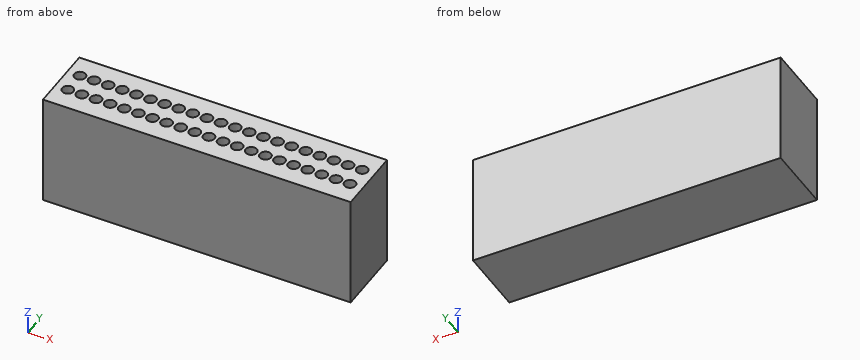
```python
from build123d import *

# Parameters (mm, degrees)
SKETCH2_W           = 27.25
SKETCH2_H           = 6
BOSS_EXTRUDE1_DEPTH = 10
SKETCH3_R           = 0.5
CUT_EXTRUDE1_DEPTH  = 5


with BuildPart() as part:
    # Sketch2 → Boss-Extrude1 (new body)
    with BuildSketch(Plane.XY):
        with Locations((13.625, 3)):
            Rectangle(SKETCH2_W, SKETCH2_H)
    extrude(amount=BOSS_EXTRUDE1_DEPTH)

    # Sketch3 → Cut-Extrude1 (cut)
    with BuildSketch(Plane.XY.offset(10)):
        with Locations((1.125, 2)):
            Circle(SKETCH3_R)
        with Locations((2.375, 2)):
            Circle(SKETCH3_R)
        with Locations((3.625, 2)):
            Circle(SKETCH3_R)
        with Locations((4.875, 2)):
            Circle(SKETCH3_R)
        with Locations((6.125, 2)):
            Circle(SKETCH3_R)
        with Locations((7.375, 2)):
            Circle(SKETCH3_R)
        with Locations((8.625, 2)):
            Circle(SKETCH3_R)
        with Locations((9.875, 2)):
            Circle(SKETCH3_R)
        with Locations((11.125, 2)):
            Circle(SKETCH3_R)
        with Locations((12.375, 2)):
            Circle(SKETCH3_R)
        with Locations((13.625, 2)):
            Circle(SKETCH3_R)
        with Locations((14.875, 2)):
            Circle(SKETCH3_R)
        with Locations((16.125, 2)):
            Circle(SKETCH3_R)
        with Locations((17.375, 2)):
            Circle(SKETCH3_R)
        with Locations((18.625, 2)):
            Circle(SKETCH3_R)
        with Locations((19.875, 2)):
            Circle(SKETCH3_R)
        with Locations((21.125, 2)):
            Circle(SKETCH3_R)
        with Locations((22.375, 2)):
            Circle(SKETCH3_R)
        with Locations((23.625, 2)):
            Circle(SKETCH3_R)
        with Locations((24.875, 2)):
            Circle(SKETCH3_R)
        with Locations((26.125, 2)):
            Circle(SKETCH3_R)
    cut_extrude1 = extrude(amount=-CUT_EXTRUDE1_DEPTH, mode=Mode.SUBTRACT)

    # Mirror1: Cut-Extrude1 across plane
    add(cut_extrude1.mirror(Plane(origin=(0, 3, 0), x_dir=(0, 0, 1), z_dir=(0, -1, 0))), mode=Mode.SUBTRACT)


solid = part.part
```
Build history of the part. All positions in model axes, mm. Round coordinates to 2 decimals unless told otherwise and drop trailing zeros. Write each loop counter-clockwise with the first axis right and the second up, starting at its lowest first coordinate (ties: lowest second). Pieces come first, ordered by that corner, then holes. Notation, with made-up numbers: (-28.75, 80) -> (11.25, 80) arc R23 ccw to (11.25, 108) -> close; hole circle Ø6 at (88.25, 24.25). An arc over 180 degrees is marked (long way). Put each result on its own line as item: value.
Item 1: Flat gauge pin, fed straight in: P1, Ø0.5, axis at x = 20, y = 2, coming from the +Z side. Where does the tip first touch, or does it go through?
Here are the results:
P1: stops at z = 5
Item 2: Slice it at A-A, the plane x = 25. Give the cut face in (y, z), plus the area to 3 significant figures.
Here are the results:
outline: (0, 0) -> (6, 0) -> (6, 10) -> (4.48, 10) -> (4.48, 5) -> (3.52, 5) -> (3.52, 10) -> (2.48, 10) -> (2.48, 5) -> (1.52, 5) -> (1.52, 10) -> (0, 10) -> close
area: 50.3 mm^2
Item 3: Wall check: probe 1 along Y at (x, z) = (11.5, 7.25); probe 2 along Y at (x, z) = (7.5, 6.25); probe 3 along Z at (x, y) = (4.75, 3.9). Give the ranges that are in metal, low to high. Write a range as from..to.
Here are the results:
probe 1: y = 0..1.67, 2.33..3.67, 4.33..6
probe 2: y = 0..1.52, 2.48..3.52, 4.48..6
probe 3: z = 0..5
Item 4: Slice it at B-B, the plane z = 8. Count the separate pieces of the cut face and the enclosed holes in it, plus the area to 3 significant figures.
Here are the results:
separate pieces: 1
enclosed holes: 42
area: 131 mm^2
